```python
from build123d import *

# Parameters (mm, degrees)
SKETCH1_W                            = 70
SKETCH1_H                            = 70
BOSS_EXTRUDE1_DEPTH                  = 9.525
CBORE_FOR_M5_SHCS2_AT_2_COUNT        = 2
CBORE_FOR_M5_SHCS2_AT_2_PITCH        = 13.393920133
CBORE_FOR_M5_SHCS2_AT_3_COUNT        = 2
CBORE_FOR_M5_SHCS2_AT_3_PITCH        = 24.748737342
CBORE_FOR_M5_SHCS2_AT_4_COUNT        = 2
CBORE_FOR_M5_SHCS2_AT_4_PITCH        = 32.335783638
CBORE_FOR_M5_SHCS2_AT_5_COUNT        = 2
CBORE_FOR_M5_SHCS2_AT_5_PITCH        = 35
CBORE_FOR_M5_SHCS2_AT_6_COUNT        = 2
CBORE_FOR_M5_SHCS2_AT_6_PITCH        = 32.335783638
CBORE_FOR_M5_SHCS2_AT_7_COUNT        = 2
CBORE_FOR_M5_SHCS2_AT_7_PITCH        = 24.748737342
CBORE_FOR_M5_SHCS2_AT_8_COUNT        = 2
CBORE_FOR_M5_SHCS2_AT_8_PITCH        = 13.393920133
TAP_DRILL_FOR_M4X0_7_TAP1_AT_2_COUNT = 2
TAP_DRILL_FOR_M4X0_7_TAP1_AT_2_PITCH = 25
SKETCH9_R                            = 7.5
CUT_EXTRUDE1_DEPTH                   = 51.405611047
CBORE_FOR_M4_SHCS1_AT_2_COUNT        = 2
CBORE_FOR_M4_SHCS1_AT_2_PITCH        = 40
FILLET1_R                            = 15


with BuildPart() as part:
    # Sketch1 → Boss-Extrude1 (new body)
    with BuildSketch(Plane(origin=(0, 0, 0), x_dir=(1, 0, 0), z_dir=(0, 1, 0))):
        Rectangle(SKETCH1_W, SKETCH1_H)
    extrude(amount=BOSS_EXTRUDE1_DEPTH)

    # Sketch4 → CBORE for M5 SHCS2 (revolve, cut)
    with BuildSketch(Plane(origin=(0, 0, 22.5), x_dir=(0, 0, -1), z_dir=(1, 0, 0))):
        Polygon((0, 0), (0, 9.525), (2.75, 9.525), (2.75, 5), (5, 5), (5, 0.025), (5.025, 0), align=None)
    cbore_for_m5_shcs2 = revolve(axis=Axis((0, -6.35, 22.5), (0, 1, 0)), mode=Mode.SUBTRACT)

    # CBORE for M5 SHCS2 at 2: CBORE for M5 SHCS2 ×2
    with Locations(*[Vector(0.9238795325112866, 0, -0.38268343236509006) * (i * CBORE_FOR_M5_SHCS2_AT_2_PITCH) for i in range(1, CBORE_FOR_M5_SHCS2_AT_2_COUNT)]):
        add(cbore_for_m5_shcs2, mode=Mode.SUBTRACT)

    # CBORE for M5 SHCS2 at 3: CBORE for M5 SHCS2 ×2
    with Locations(*[Vector(0.7071067811865475, 0, -0.7071067811865477) * (i * CBORE_FOR_M5_SHCS2_AT_3_PITCH) for i in range(1, CBORE_FOR_M5_SHCS2_AT_3_COUNT)]):
        add(cbore_for_m5_shcs2, mode=Mode.SUBTRACT)

    # CBORE for M5 SHCS2 at 4: CBORE for M5 SHCS2 ×2
    with Locations(*[Vector(0.3826834323650898, 0, -0.9238795325112868) * (i * CBORE_FOR_M5_SHCS2_AT_4_PITCH) for i in range(1, CBORE_FOR_M5_SHCS2_AT_4_COUNT)]):
        add(cbore_for_m5_shcs2, mode=Mode.SUBTRACT)

    # CBORE for M5 SHCS2 at 5: CBORE for M5 SHCS2 ×2
    with Locations(*[(0, 0, -i * CBORE_FOR_M5_SHCS2_AT_5_PITCH) for i in range(1, CBORE_FOR_M5_SHCS2_AT_5_COUNT)]):
        add(cbore_for_m5_shcs2, mode=Mode.SUBTRACT)

    # CBORE for M5 SHCS2 at 6: CBORE for M5 SHCS2 ×2
    with Locations(*[Vector(-0.3826834323650896, 0, -0.9238795325112868) * (i * CBORE_FOR_M5_SHCS2_AT_6_PITCH) for i in range(1, CBORE_FOR_M5_SHCS2_AT_6_COUNT)]):
        add(cbore_for_m5_shcs2, mode=Mode.SUBTRACT)

    # CBORE for M5 SHCS2 at 7: CBORE for M5 SHCS2 ×2
    with Locations(*[Vector(-0.7071067811865474, 0, -0.7071067811865477) * (i * CBORE_FOR_M5_SHCS2_AT_7_PITCH) for i in range(1, CBORE_FOR_M5_SHCS2_AT_7_COUNT)]):
        add(cbore_for_m5_shcs2, mode=Mode.SUBTRACT)

    # CBORE for M5 SHCS2 at 8: CBORE for M5 SHCS2 ×2
    with Locations(*[Vector(-0.9238795325112867, 0, -0.38268343236509) * (i * CBORE_FOR_M5_SHCS2_AT_8_PITCH) for i in range(1, CBORE_FOR_M5_SHCS2_AT_8_COUNT)]):
        add(cbore_for_m5_shcs2, mode=Mode.SUBTRACT)

    # Sketch8 → Tap Drill for M4x0.7 Tap1 (revolve, cut)
    with BuildSketch(Plane(origin=(35, 4.5, 0), x_dir=(0, 0, -1), z_dir=(0, 1, 0))):
        Polygon((0, 0), (0, 8.991420021), (1.65, 8), (1.65, 0.025), (1.675, 0), align=None)
    tap_drill_for_m4x0_7_tap1 = revolve(axis=Axis((41.35, 4.5, 0), (-1, 0, 0)), mode=Mode.SUBTRACT)

    # Tap Drill for M4x0.7 Tap1 at 2: Tap Drill for M4x0.7 Tap1 ×2
    with Locations(*[(0, 0, -i * TAP_DRILL_FOR_M4X0_7_TAP1_AT_2_PITCH) for i in range(1, TAP_DRILL_FOR_M4X0_7_TAP1_AT_2_COUNT)]):
        add(tap_drill_for_m4x0_7_tap1, mode=Mode.SUBTRACT)

    # Sketch9 → Cut-Extrude1 (cut, through all)
    with BuildSketch(Plane.XZ):
        with Locations(Location((0, 5, 0), (0, 0, 270))):
            Circle(SKETCH9_R)
    extrude(amount=-CUT_EXTRUDE1_DEPTH, mode=Mode.SUBTRACT)

    # Sketch15 → CBORE for M4 SHCS1 (revolve, cut)
    with BuildSketch(Plane(origin=(-20, 9.525, -30.2375), x_dir=(0, 0, 1), z_dir=(1, 0, 0))):
        Polygon((0, 0), (0, 9.525), (2.25, 9.525), (2.25, 4), (4, 4), (4, 0.025), (4.025, 0), align=None)
    cbore_for_m4_shcs1 = revolve(axis=Axis((-20, 15.875, -30.2375), (0, -1, 0)), mode=Mode.SUBTRACT)

    # CBORE for M4 SHCS1 at 2: CBORE for M4 SHCS1 ×2
    with Locations(*[(i * CBORE_FOR_M4_SHCS1_AT_2_PITCH, 0, 0) for i in range(1, CBORE_FOR_M4_SHCS1_AT_2_COUNT)]):
        add(cbore_for_m4_shcs1, mode=Mode.SUBTRACT)

    # Mirror1: Tap Drill for M4x0.7 Tap1 across plane
    add(tap_drill_for_m4x0_7_tap1.mirror(Plane(origin=(0, 0, 0), x_dir=(0, 0, 1), z_dir=(1, 0, 0))), mode=Mode.SUBTRACT)

    # Mirror1 copy 1 sketch → Mirror1 copy 1 (revolve, cut)
    with BuildSketch(Plane(origin=(-35, 4.5, -25), x_dir=(0, 0, -1), z_dir=(0, 1, 0))):
        Polygon((0, 0), (0, -8.991420021), (1.65, -8), (1.65, -0.025), (1.675, 0), align=None)
    revolve(axis=Axis((-41.35, 4.5, -25), (-1, 0, 0)), mode=Mode.SUBTRACT)

    # Fillet1
    fillet1_edges = [part.edges().sort_by_distance(p)[0] for p in [
        (35, 4.7625, 35),
        (-35, 4.7625, 35),
    ]]
    fillet(fillet1_edges, radius=FILLET1_R)


solid = part.part
```
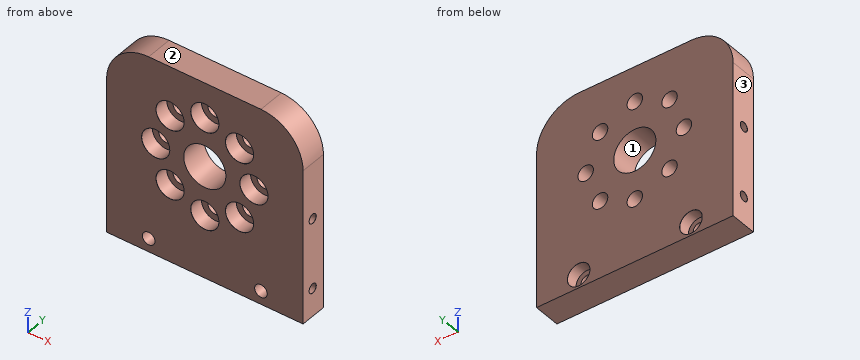
The model under review builds one solid part; all positions refer to its coordinate system, in mm. Face numbers are marked on the shaded views. Round coordinates to 2 decimals unless told otherwise and drop trailing zeros. Write each loop counter-clockwise with the first axis right and the second up, starting at its lowest first coordinate (ties: lowest second). Pieces come first, ordered by that corner, then holes. Notation, with made-up numbers: (-6, -22.5) - (30, -22.5) arc R15 ccw to (30, 2.5) - close; hole circle Ø9 at (40.5, 23.5). An arc over 180 degrees is marked (long way). Use one line per item in the form item = value.
Q1. For line 1 (X direction, y = 1.75, z = -7); line 2 (Z direction, x = 31.5, y = 4.5); line 3 (X direction, y = 3.5, z = -6), list the stretches that pass through material, from the lowest coordinate up. Write a range as [from, to].
Answer key:
line_1 = [-35, -17.36], [-7.39, 7.39], [17.36, 35]
line_2 = [-35, -26.65], [-23.35, -1.65], [1.65, 29.63]
line_3 = [-35, -17.18], [-7.57, 7.57], [17.18, 35]
Q2. Insertion check: pin 1 Ø6.5 at (x, z) = (12.37, -7.37) entering from -Y; pin 2 Ø1 at (y, z) = (4.5, -25) entering from +X; pin 3 Ø2.5 at (y, z) = (4.5, -25) entering from -X. Each pin has a flat end and moves straight along its axis. Give the tip position at first contact, or say it passes through.
Answer key:
pin_1 = 5
pin_2 = 26.31
pin_3 = -26.76
Q3. Consider section A-A (x = -6). State the section outline as (y, z) points (3 decimals), and give its area (3 significant figures).
Answer key:
outline = (0, -35) - (9.525, -35) - (9.525, 0.5) - (0, 0.5) - close; (0, 9.5) - (9.525, 9.5) - (9.525, 35) - (0, 35) - close
area = 581 mm2
Q4. Draft analysis for pull direction Z (two halves, no side actions). For the marked faces 1, 2 and 3, state which applies: +Z half, -Z half, draft (parallel to the pull), parting line (faces both ways), or undercut.
Answer key:
face_1 = undercut
face_2 = +Z half
face_3 = draft
Q5. Consider section B-B (x = -19). State how many separate pieces and enclosed holes the cut face has, and give its area (3 significant figures).
Answer key:
separate_pieces = 3
enclosed_holes = 0
area = 545 mm2
